The model under review builds one solid part; all positions refer to its coordinate system, in mm. A direction names the side the tool comes from. Coordinates: 2 decimals unless noted, no trailing zeros. Order: outer loops, then holes, each group sorted by start corner. A loop starts at its lowest first (then second) coordinate and runs counter-clockwise, first axis right, second up. Notation, with made-up numbers: M 69.5,17 L 116.5,17 A27 cw 116.5,50 Z; hole C 71,7 d7. An arc over 180 degrees is marked long. One line per item, written item: value.
```python
from build123d import *

# Parameters (mm, degrees)
SKETCH1_W           = 107.95
SKETCH1_H           = 31.75
BOSS_EXTRUDE1_DEPTH = 31.75
SKETCH3_W           = 63.5
SKETCH3_H           = 76.2
SKETCH3_R           = 3.429
BOSS_EXTRUDE2_DEPTH = 6.35
FILLET1_R           = 5.08


with BuildPart() as part:
    # Sketch1 → Boss-Extrude1 (new, symmetric)
    with BuildSketch(Plane(origin=(0, 0, 0), x_dir=(0, 0, -1), z_dir=(1, 0, 0))):
        Rectangle(SKETCH1_W, SKETCH1_H)
    extrude(amount=BOSS_EXTRUDE1_DEPTH, both=True)

    # Sketch2 → Cut-Revolve1 (revolve, cut)
    with BuildSketch(Plane(origin=(0, 0, 0), x_dir=(0, 0, -1), z_dir=(1, 0, 0))):
        Polygon((30.787113889, -1.024256513), (21.709471638, -34.902478605), (-1.905, -28.575), (15.934173595, 38.001702221), (59.482939473, 26.332845573), (50.721408129, -6.365634557), align=None)
    revolve(axis=Axis((0, -21.465443212, 0), (0, 0.9659258262890701, -0.2588190451025143)), mode=Mode.SUBTRACT)

    # Sketch3 → Boss-Extrude2 (add)
    with BuildSketch(Plane.XY.offset(53.975)):
        Rectangle(SKETCH3_W, SKETCH3_H)
        with Locations((-19.05, 25.4)):
            Circle(SKETCH3_R, mode=Mode.SUBTRACT)
        with Locations((-6.35, 25.4)):
            Circle(SKETCH3_R, mode=Mode.SUBTRACT)
        with Locations((6.35, 25.4)):
            Circle(SKETCH3_R, mode=Mode.SUBTRACT)
        with Locations((19.05, 25.4)):
            Circle(SKETCH3_R, mode=Mode.SUBTRACT)
        with Locations((-6.35, -25.4)):
            Circle(SKETCH3_R, mode=Mode.SUBTRACT)
        with Locations((6.35, -25.4)):
            Circle(SKETCH3_R, mode=Mode.SUBTRACT)
        with Locations((19.05, -25.4)):
            Circle(SKETCH3_R, mode=Mode.SUBTRACT)
        with Locations((-19.05, -25.4)):
            Circle(SKETCH3_R, mode=Mode.SUBTRACT)
    extrude(amount=BOSS_EXTRUDE2_DEPTH)

    # Fillet1
    fillet1_edges = [part.edges().sort_by_distance(p)[0] for p in [
        (0, 15.875, 53.975),
        (0, -15.875, 53.975),
    ]]
    fillet(fillet1_edges, radius=FILLET1_R)


solid = part.part
```
(1) We need section C-C, the plane x = 6.35. State the section outline as (y, z) points (3 decimals).
Geometry results:
outline: M -38.1,53.975 L -28.829,53.975 L -28.829,60.325 L -38.1,60.325 Z; M -21.971,53.975 L -20.955,53.975 A5.08 cw -15.875,48.895 L -15.875,22.943 L 11.414,15.631 L 15.875,32.282 L 15.875,48.895 A5.08 cw 20.955,53.975 L 21.971,53.975 L 21.971,60.325 L -21.971,60.325 Z; M -15.875,-53.975 L 7.513,-53.975 L -6.249,-50.287 L -0.807,-29.977 L -15.875,-25.939 Z; M 28.829,53.975 L 38.1,53.975 L 38.1,60.325 L 28.829,60.325 Z
(2) For L1, parallel to X at y = -25, z = 56; L2, parallel to Y at x = 19.05, z = 59; L3, parallel to X at y = -1, z = -4.5, list the stretches that pass through material, from the lowest coordinate up.
Geometry results:
L1: x = -31.75 to -22.46, -15.64 to -9.76, -2.94 to 2.94, 9.76 to 15.64, 22.46 to 31.75
L2: y = -38.1 to -28.83, -21.97 to 21.97, 28.83 to 38.1
L3: x = -31.75 to -24.43, 24.43 to 31.75
(3) Tool access review of faces 4 (the cylindrical face through (-28.63, 14.94, 26.3)), 5 (the flat face through (0, -38.1, 57)), 6 (the flat face through (0, 30, 53.975)), 7 (the cylindrical face through (-17.468, 22.358, 57.106)), 8 (the flat face through (0, -29, 53.975)): name each direction out of +Z, -Z, +X, -X, +Y, -Y from which nothing blocks a thin tool from reaching the whole face with its end or side.
Geometry results:
face 4: none
face 5: +Z, -Z, +X, -X, -Y
face 6: -Z, +X, -X, +Y
face 7: +Z, -Z
face 8: -Z, +X, -X, -Y
(4) We need section A-A, the plane y = -25.4. State the section outline as (x, z) points (3 decimals).
Geometry results:
outline: M -31.75,53.975 L -22.479,53.975 L -22.479,60.325 L -31.75,60.325 Z; M -15.621,53.975 L -9.779,53.975 L -9.779,60.325 L -15.621,60.325 Z; M -2.921,53.975 L 2.921,53.975 L 2.921,60.325 L -2.921,60.325 Z; M 9.779,53.975 L 15.621,53.975 L 15.621,60.325 L 9.779,60.325 Z; M 22.479,53.975 L 31.75,53.975 L 31.75,60.325 L 22.479,60.325 Z
(5) We need section D-D, the plane z = 43. State the section outline as (x, y) points (3 decimals).
Geometry results:
outline: M -31.75,-15.875 L 31.75,-15.875 L 31.75,15.875 L -31.75,15.875 Z
(6) Insertion check: pin 1 Ø13.5 at (x, y) = (5.5, 32) entering from -Z (3 decimals); pin 2 Ø6 at (x, y) = (-19.05, -25.4) entering from +Z; pin 3 Ø12 at (x, z) = (22, -49) entering from +Y (3 decimals); pin 4 Ø12 at (x, z) = (-7.5, 21.5) entering from +Y. Each pin has a flat end and moves straight along its axis. Give the tip position at first contact, or say it passes through.
Geometry results:
pin 1: stops at z = 53.975
pin 2: passes through
pin 3: stops at y = 15.875
pin 4: stops at y = 14.59
(7) We need section B-B, the plane x = -13.5. State the section outline as (y, z) points (1 decimal).
Geometry results:
outline: M -38.1,54 L -21,54 A5.1 cw -15.9,48.9 L -15.9,19.6 L 10.6,12.5 L 15.9,32.3 L 15.9,48.9 A5.1 cw 21,54 L 38.1,54 L 38.1,60.3 L -38.1,60.3 Z; M -15.9,-54 L 13.8,-54 L -5.8,-48.7 L 0,-26.9 L -15.9,-22.6 Z
(8) Mouldability with a two-part tool opening along X and no side actions: class faces 1 (the cylindrical face through (-7.09, -28.75, 57.11)), 2 (the flat face through (31.75, -3, 11)), 3 (the cylindrical face through (0.444, -17.403, 52.526)) as +X half, -X half, draft (parallel to the pull), parting line (faces both ways), or undercut.
Geometry results:
face 1: undercut
face 2: +X half
face 3: draft
